Can you work these out from the model? Positions are in its coordinate system, mm. Give positions to 0.01 mm unless a question says otherwise; leave off trailing zeros. Order: outer loops, then holes, each group sorted by start corner. A loop starts at its lowest first (then second) coordinate and runs counter-clockwise, first axis right, second up. Notation, with made-up numbers: (-24, 18.5) - (10, 18.5) arc R26 cw to (10, 47.5) - close; hole circle Ø10 at (-2.75, 71.5). An arc over 180 degrees is marked (long way). Use one line per item in the form item = value. Start each with the question number.
1) Suppose I cut it at C-C, the plane x = 12.7. Write out the boundary of the cut face in (y, z) (3 decimals).
2) Suppose I cut it at D-D, the plane y = 1. Write out the boundary of the cut face in (x, z) (3 decimals).
3) Suppose I cut it at B-B, the plane y = 27. Write out the boundary of the cut face in (x, z) (3 decimals), and give its area (3 significant figures).
4) Suppose I cut it at A-A, the plane x = -63.5. Write out the boundary of the cut face in (y, z) (3 decimals).
5) Please list where these lines run through material, in increasing order: probe 1 along X at (y, z) = (-6.5, 1); probe 2 along Y at (x, z) = (0, 0.25); probe 3 along Y at (x, z) = (12.5, -0.75).
6) For pin 1 (3 mm diameter, centred on y = 29, z = 0, fed in from -X); pin 2 (5.5 mm diameter, centred on x = 50.8, y = -12.7, fed in from +Z) (3 decimals); pin 3 (1.9 mm diameter, centred on x = -72, z = -1, fed in from +Y); pin 4 (3.5 mm diameter, centred on x = -25.4, y = -12.7, fed in from -Z), each with a flat end and sliding along its axis, tell me the tip position at first contact or that it passes through.
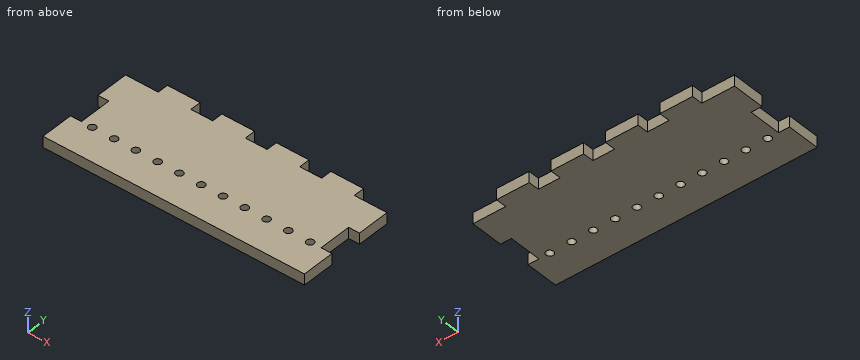
```python
from build123d import *

# Parameters (mm, degrees)
SKETCH1_W            = 152.4
SKETCH1_H            = 63.5
BOSS_EXTRUDE1_DEPTH  = 3.175
SKETCH2_R            = 2.159
CUT_EXTRUDE1_DEPTH   = 83.793870546
LPATTERN1_COUNT      = 11
LPATTERN1_PITCH      = 12.7
LPATTERN1_COUNT_DIR2 = 11
LPATTERN1_PITCH_DIR2 = 12.7
SKETCH3_W            = 19.05
SKETCH3_H            = 6.35
CUT_EXTRUDE2_DEPTH   = 83.793870546
SKETCH4_W            = 12.7
SKETCH4_H            = 6.35
CUT_EXTRUDE3_DEPTH   = 83.793870546
LPATTERN2_COUNT      = 3
LPATTERN2_PITCH      = 31.75
SKETCH5_W            = 6.35
SKETCH5_H            = 19.05
CUT_EXTRUDE4_DEPTH   = 83.793870546


with BuildPart() as part:
    # Sketch1 → Boss-Extrude1 (new, symmetric)
    with BuildSketch(Plane.XY):
        Rectangle(SKETCH1_W, SKETCH1_H)
    extrude(amount=BOSS_EXTRUDE1_DEPTH, both=True)

    # Sketch2 → Cut-Extrude1 (cut, through all)
    with BuildSketch(Plane(origin=(0, 0, -3.175), x_dir=(-1, 0, 0), z_dir=(0, 0, -1))):
        with Locations((0, -12.7)):
            Circle(SKETCH2_R)
    cut_extrude1 = extrude(amount=-CUT_EXTRUDE1_DEPTH, mode=Mode.SUBTRACT)

    # LPattern1: Cut-Extrude1 11 × 11, 10 skipped
    with Locations(*[Vector(-1, 0, 0) * (i * LPATTERN1_PITCH) + Vector(1, 0, 0) * (j * LPATTERN1_PITCH_DIR2) for i in range(LPATTERN1_COUNT) for j in range(LPATTERN1_COUNT_DIR2) if (i, j) not in ((0, 0), (0, 6), (1, 7), (2, 8), (3, 9), (4, 10), (6, 0), (7, 1), (8, 2), (9, 3), (10, 4))]):
        add(cut_extrude1, mode=Mode.SUBTRACT)

    # Sketch3 → Cut-Extrude2 (cut, through all)
    with BuildSketch(Plane(origin=(0, 0, -3.175), x_dir=(-1, 0, 0), z_dir=(0, 0, -1))):
        with Locations((-66.675, 28.575)):
            Rectangle(SKETCH3_W, SKETCH3_H)
    cut_extrude2 = extrude(amount=-CUT_EXTRUDE2_DEPTH, mode=Mode.SUBTRACT)

    # Mirror1: Cut-Extrude2 across plane
    add(cut_extrude2.mirror(Plane(origin=(0, 0, 0), x_dir=(0, 0, 1), z_dir=(1, 0, 0))), mode=Mode.SUBTRACT)

    # Sketch4 → Cut-Extrude3 (cut, through all)
    with BuildSketch(Plane(origin=(0, 0, -3.175), x_dir=(-1, 0, 0), z_dir=(0, 0, -1))):
        with Locations((-31.75, 28.575)):
            Rectangle(SKETCH4_W, SKETCH4_H)
    cut_extrude3 = extrude(amount=-CUT_EXTRUDE3_DEPTH, mode=Mode.SUBTRACT)

    # LPattern2: Cut-Extrude3 ×3
    with Locations(*[(-i * LPATTERN2_PITCH, 0, 0) for i in range(1, LPATTERN2_COUNT)]):
        add(cut_extrude3, mode=Mode.SUBTRACT)

    # Sketch5 → Cut-Extrude4 (cut, through all)
    with BuildSketch(Plane(origin=(0, 0, -3.175), x_dir=(-1, 0, 0), z_dir=(0, 0, -1))):
        with Locations((-73.025, -3.175)):
            Rectangle(SKETCH5_W, SKETCH5_H)
    cut_extrude4 = extrude(amount=-CUT_EXTRUDE4_DEPTH, mode=Mode.SUBTRACT)

    # Mirror2: Cut-Extrude4 across plane
    add(cut_extrude4.mirror(Plane(origin=(0, 0, 0), x_dir=(0, 0, 1), z_dir=(1, 0, 0))), mode=Mode.SUBTRACT)


solid = part.part
```
Result sheet:
q1.outline = (-31.75, -3.175) - (-14.859, -3.175) - (-14.859, 3.175) - (-31.75, 3.175) - close; (-10.541, -3.175) - (31.75, -3.175) - (31.75, 3.175) - (-10.541, 3.175) - close
q2.outline = (-69.85, -3.175) - (69.85, -3.175) - (69.85, 3.175) - (-69.85, 3.175) - close
q3.outline = (-57.15, -3.175) - (-38.1, -3.175) - (-38.1, 3.175) - (-57.15, 3.175) - close; (-25.4, -3.175) - (-6.35, -3.175) - (-6.35, 3.175) - (-25.4, 3.175) - close; (6.35, -3.175) - (25.4, -3.175) - (25.4, 3.175) - (6.35, 3.175) - close; (38.1, -3.175) - (57.15, -3.175) - (57.15, 3.175) - (38.1, 3.175) - close
q3.area = 484 mm²
q4.outline = (-31.75, -3.175) - (-14.859, -3.175) - (-14.859, 3.175) - (-31.75, 3.175) - close; (-10.541, -3.175) - (25.4, -3.175) - (25.4, 3.175) - (-10.541, 3.175) - close
q5.probe_1 = -69.85 to 69.85
q5.probe_2 = -31.75 to -14.86, -10.54 to 25.4
q5.probe_3 = -31.75 to -14.85, -10.55 to 31.75
q6.pin_1 = -57.15
q6.pin_2 = 3.175
q6.pin_3 = 25.4
q6.pin_4 = through
